Verification items for the finished model (mm, model axes). A direction names the side the tool comes from. Round coordinates to 2 decimals unless told otherwise and drop trailing zeros. Write each loop counter-clockwise with the first axis right and the second up, starting at its lowest first coordinate (ties: lowest second). Pieces come first, ordered by that corner, then holes. Notation, with made-up numbers: (68, 12) - (95, 12) arc R26 cw to (95, 46) - close; hole circle Ø10 at (-9, 24.25). An arc over 180 degrees is marked (long way). Answer as a JSON object with one key per item and string values.
```python
from build123d import *

# Parameters (mm, degrees)
F0_R     = 1
F0_R_2   = 7.5
F0_R_3   = 2
F1_DEPTH = 30
F2_DEPTH = 3.5
F3_DEPTH = 15
F4_DEPTH = 1.5


with BuildPart() as f1:
    # F0 (on Top) → F1 (new body)
    with BuildSketch(Plane.XY):
        with BuildLine():
            ThreePointArc((10, 9), (9.7071067812, 9.7071067812), (9, 10))
            Line((9, 10), (-9, 10))
            ThreePointArc((-9, 10), (-9.7071067812, 9.7071067812), (-10, 9))
            Line((-10, 9), (-10, -9))
            ThreePointArc((-10, -9), (-9.7071067812, -9.7071067812), (-9, -10))
            Line((-9, -10), (9, -10))
            ThreePointArc((9, -10), (9.7071067812, -9.7071067812), (10, -9))
            Line((10, -9), (10, 9))
        make_face()
        with Locations((-8, -8)):
            Circle(F0_R, mode=Mode.SUBTRACT)
        with Locations((8, -8)):
            Circle(F0_R, mode=Mode.SUBTRACT)
        with Locations((-8, 8)):
            Circle(F0_R, mode=Mode.SUBTRACT)
        Circle(F0_R_2, mode=Mode.SUBTRACT)
        with Locations((8, 8)):
            Circle(F0_R, mode=Mode.SUBTRACT)
        Circle(F0_R_2)
        Circle(F0_R_3, mode=Mode.SUBTRACT)
        Circle(F0_R_3)
        with Locations((-8, -8)):
            Circle(F0_R)
        with Locations((8, 8)):
            Circle(F0_R)
        with Locations((8, -8)):
            Circle(F0_R)
        with Locations((-8, 8)):
            Circle(F0_R)
    extrude(amount=-F1_DEPTH)

    # F0 (on Top) → F2 (cut)
    with BuildSketch(Plane.XY):
        with Locations((-8, 8)):
            Circle(F0_R)
        with Locations((8, 8)):
            Circle(F0_R)
        with Locations((-8, -8)):
            Circle(F0_R)
        with Locations((8, -8)):
            Circle(F0_R)
    extrude(amount=-F2_DEPTH, mode=Mode.SUBTRACT)

    # F0 (on Top) → F3 (join)
    with BuildSketch(Plane.XY):
        Circle(F0_R_3)
    extrude(amount=F3_DEPTH)

    # F0 (on Top) → F4 (join)
    with BuildSketch(Plane.XY):
        Circle(F0_R_2)
        Circle(F0_R_3, mode=Mode.SUBTRACT)
    extrude(amount=F4_DEPTH)


solid = f1.part
```
Q1. Gauge pin test, flat ends, axial feed: P1, Ø1, axis at x = -2.5, y = -4, coming from the +Z side; P2, Ø1.5, axis at x = 0.5, z = 3, coming from the +Y side; P3, Ø1.6, axis at x = 8, y = -8, coming from the +Z side; P4, Ø2, axis at x = -4.5, z = 6, coming from the -Y side. Record the tip position at first contact, or that the pin passes through.
Geometry check:
{"P1": "stops at z = 1.5", "P2": "stops at y = 2", "P3": "stops at z = -3.5", "P4": "passes through"}
Q2. Section check D-D, the plane y = -6. Record the cut outline in (x, z).
Geometry check:
{"outline": "(-10, -30) - (10, -30) - (10, 0) - (4.5, 0) - (4.5, 1.5) - (-4.5, 1.5) - (-4.5, 0) - (-10, 0) - close"}
Q3. Section check A-A, the plane y = 0. Record the cut outline in (x, z).
Geometry check:
{"outline": "(-10, -30) - (10, -30) - (10, 0) - (7.5, 0) - (7.5, 1.5) - (2, 1.5) - (2, 15) - (-2, 15) - (-2, 1.5) - (-7.5, 1.5) - (-7.5, 0) - (-10, 0) - close"}
Q4. Release check for a two-part mould opening along Y. For faces 1 (the cylindrical face through (9.699, -9.715, -14.79)), 2 (the flat face through (8, 8, -3.5)), 3 (the flat face through (0, 10, -15)) record: released by +Y, released by -Y, zero draft, split by the parting line, or undercut.
Geometry check:
{"face 1": "released by -Y", "face 2": "undercut", "face 3": "released by +Y"}
Q5. Section check B-B, the plane x = 8. Record the cut outline in (y, z).
Geometry check:
{"outline": "(-10, -30) - (10, -30) - (10, 0) - (9, 0) - (9, -3.5) - (7, -3.5) - (7, 0) - (-7, 0) - (-7, -3.5) - (-9, -3.5) - (-9, 0) - (-10, 0) - close"}
Q6. Set-up check for faces 4 (the flat face through (-8, -8, -3.5)), 5 (the flat face through (0, 0, -30)): record each of +Z, -Z, +X, -X, +Y, -Y from which the full face is reachable in a straight line by a thin tool's end or side.
Geometry check:
{"face 4": "+Z", "face 5": "-Z, +X, -X, +Y, -Y"}
Q7. Material ranges on line 1 along Y through (x, z) = (8, -0.95); line 2 along Z through (x, y) = (-7.25, -4); line 3 along Z through (x, y) = (2, 2.5), recorded low to high. Write a range as [from, to].
Geometry check:
{"line 1": "y = [-10, -9], [-7, 7], [9, 10]", "line 2": "z = [-30, 0]", "line 3": "z = [-30, 1.5]"}
Q8. Section check C-C, the plane z = 6.5. Record the cut outline in (x, y), then the cut area to 3 significant figures.
Geometry check:
{"outline": "circle Ø4 at (0, 0)", "area": "12.6 mm2"}
